Input: part model. Units: mm. Frame: model coordinates. A direction names the side the tool comes from. Coordinates: 2 decimals unless noted, no trailing zeros. Order: outer loops, then holes, each group sorted by start corner. A loop starts at its lowest first (then second) coordinate and runs counter-clockwise, first axis right, second up. Notation, with made-up numbers: (1.5, 88.25) -> (58.5, 88.25) arc R18 cw to (58.5, 120.25) -> close; hole circle Ø1 at (-23.75, 85.25). An arc over 180 degrees is marked (long way). Answer as CSV lines item,"result".
from build123d import *

# Parameters (mm, degrees)
BOSS_EXTRUDE1_DEPTH      = 51
BOSS_EXTRUDE1_DEPTH_BACK = 51
SKETCH2_W                = 3
SKETCH2_H                = 78.95
BOSS_EXTRUDE2_DEPTH      = 102
SKETCH3_W                = 5
SKETCH3_H                = 39
SKETCH3_W_2              = 3
BOSS_EXTRUDE3_DEPTH      = 102
SKETCH4_W                = 55
SKETCH4_H                = 39
BOSS_EXTRUDE4_DEPTH      = 1
BOSS_EXTRUDE5_DEPTH      = 1.75
SKETCH7_R                = 1.8
CUT_EXTRUDE1_DEPTH       = 6


with BuildPart() as part:
    # Sketch1 → Boss-Extrude1 (new, two sides: drawn at the far end of the back side and taken through both)
    with BuildSketch(Plane.XY.offset(-BOSS_EXTRUDE1_DEPTH_BACK)):
        Polygon((24.362132034, 0), (24.362132034, 121), (27.362132034, 121), (27.362132034, 111), (87.362132034, 111), (87.362132034, 108), (27.362132034, 108), (27.362132034, 78), (87.362132034, 78), (87.362132034, 75), (27.362132034, 75), (27.362132034, 45), (87.362132034, 45), (87.362132034, 42), (27.362132034, 42), (27.362132034, 3), (87.362132034, 3), (87.362132034, 0), align=None)
    extrude(amount=BOSS_EXTRUDE1_DEPTH + BOSS_EXTRUDE1_DEPTH_BACK)

    # Sketch2 → Boss-Extrude2 (add)
    with BuildSketch(Plane.XY.offset(51)):
        with Locations((22.862132034, 81.525)):
            Rectangle(SKETCH2_W, SKETCH2_H)
    extrude(amount=-BOSS_EXTRUDE2_DEPTH)

    # Sketch3 → Boss-Extrude3 (add)
    with BuildSketch(Plane.XY.offset(51)):
        with Locations((29.862132034, 22.5)):
            Rectangle(SKETCH3_W, SKETCH3_H)
        with Locations((65.862132034, 22.5)):
            Rectangle(SKETCH3_W_2, SKETCH3_H)
    extrude(amount=-BOSS_EXTRUDE3_DEPTH)

    # Sketch4 → Boss-Extrude4 (add)
    with BuildSketch(Plane(origin=(0, 0, -51), x_dir=(-1, 0, 0), z_dir=(0, 0, -1))):
        with Locations((-59.862132034, 22.5)):
            Rectangle(SKETCH4_W, SKETCH4_H)
    extrude(amount=-BOSS_EXTRUDE4_DEPTH)

    # Sketch5 → Boss-Extrude5 (add)
    with BuildSketch(Plane(origin=(87.362132034, 0, 0), x_dir=(0, 0, -1), z_dir=(1, 0, 0))):
        Polygon((36, 0), (36, 3), (-19, 3), (-19, 42), (-19, 75), (-19, 88), (36, 88), (36, 121), (51, 121), (51, 0), align=None)
    extrude(amount=-BOSS_EXTRUDE5_DEPTH)

    # Sketch7 → Cut-Extrude1 (cut)
    with BuildSketch(Plane.ZY.offset(-24.362132034)):
        with Locations((-29.362132034, 37)):
            Circle(SKETCH7_R)
        with Locations((-29.362132034, 10)):
            Circle(SKETCH7_R)
        with Locations((29.362132034, 10)):
            Circle(SKETCH7_R)
        with Locations((29.362132034, 37)):
            Circle(SKETCH7_R)
    extrude(amount=-CUT_EXTRUDE1_DEPTH, mode=Mode.SUBTRACT)


solid = part.part
1. Mould query, pull axis X, two halves, no side actions, for faces 6 (the face through (40, 43, 51)), 7 (the face through (30.362, 37, 29)), 8 (the face through (78, 42, 0)), 9 (the face through (85.612, 60, -16)). Classes: released by +X, released by -X, zero draft, split by the parting line, or undercut.
Findings:
face 6,"zero draft"
face 7,"released by -X"
face 8,"undercut"
face 9,"undercut"
2. Cut plane C-C (x = 71). Return the cut outline in (y, z).
Findings:
outline,"(0, -51) -> (45, -51) -> (45, 51) -> (42, 51) -> (42, -50) -> (3, -50) -> (3, 51) -> (0, 51) -> close; (75, -51) -> (78, -51) -> (78, 51) -> (75, 51) -> close; (108, -51) -> (111, -51) -> (111, 51) -> (108, 51) -> close"
3. Cut plane D-D (y = 37). Return the cut outline in (x, z), plus the area to 3 significant figures.
Findings:
outline,"(24.36, -51) -> (87.36, -51) -> (87.36, 19) -> (85.61, 19) -> (85.61, -50) -> (67.36, -50) -> (67.36, 51) -> (64.36, 51) -> (64.36, -50) -> (32.36, -50) -> (32.36, 51) -> (24.36, 51) -> (24.36, 31.16) -> (30.36, 31.16) -> (30.36, 27.56) -> (24.36, 27.56) -> (24.36, -27.56) -> (30.36, -27.56) -> (30.36, -31.16) -> (24.36, -31.16) -> close"
area,"1,250 mm2"
4. Reachability of faces 1 (the face through (30.362, 10, 29)), 2 (the face through (49, 42, 0)), 3 (the face through (85.612, 116, -44)), 4 (the face through (23, 42.05, 1)), 5 (the face through (27.362, 60, -1)) from +Z, -Z, +X, -X, +Y, -Y: full face, straight path, thin tool, end or side. Return the list, or none.
Findings:
face 1,"-X"
face 2,"+Z"
face 3,"+Z, -Z, +Y"
face 4,"+Z, -Z, -X, -Y"
face 5,"+Z, -Z"
5. Ray query, line 1 along Y through (x, z) = (58.5, 23); line 2 along Y through (x, z) = (64.5, 5); line 3 along X through (y, z) = (50, -46). Return the intervals inside material, ascending.
Findings:
line 1,"y = 0 to 3, 42 to 45, 75 to 78, 108 to 111"
line 2,"y = 0 to 45, 75 to 78, 108 to 111"
line 3,"x = 21.36 to 27.36, 85.61 to 87.36"
6. Contact query for flat-ended pins moving along their axis: pin 1 (8 mm diameter, centred on y = 37.5, z = 38.5, fed in from -X); pin 2 (6 mm diameter, centred on x = 78, z = -12.5, fed in from +Y); pin 3 (15 mm diameter, centred on y = 67, z = 22.5, fed in from +X); pin 4 (1.9 mm diameter, centred on x = 86.5, y = 84.5, fed in from +Z). Output: stop coordinate, or through.
Findings:
pin 1,"stops at x = 24.36"
pin 2,"stops at y = 111"
pin 3,"stops at x = 87.36"
pin 4,"stops at z = 19"
7. Cut plane A-A (z = -2). Return the cut outline in (x, y), plus the area to 3 significant figures.
Findings:
outline,"(21.36, 42.05) -> (24.36, 42.05) -> (24.36, 0) -> (87.36, 0) -> (87.36, 88) -> (85.61, 88) -> (85.61, 78) -> (27.36, 78) -> (27.36, 108) -> (87.36, 108) -> (87.36, 111) -> (27.36, 111) -> (27.36, 121) -> (21.36, 121) -> close; hole (27.36, 45) -> (85.61, 45) -> (85.61, 75) -> (27.36, 75) -> close; hole (32.36, 3) -> (64.36, 3) -> (64.36, 42) -> (32.36, 42) -> close; hole (67.36, 3) -> (85.61, 3) -> (85.61, 42) -> (67.36, 42) -> close"
area,"1,770 mm2"
8. Cut plane B-B (y = 54.5). Return the cut outline in (x, z), plus the area to 4 significant figures.
Findings:
outline,"(21.36, -51) -> (27.36, -51) -> (27.36, 51) -> (21.36, 51) -> close; (85.61, -51) -> (87.36, -51) -> (87.36, 19) -> (85.61, 19) -> close"
area,"734.5 mm2"
